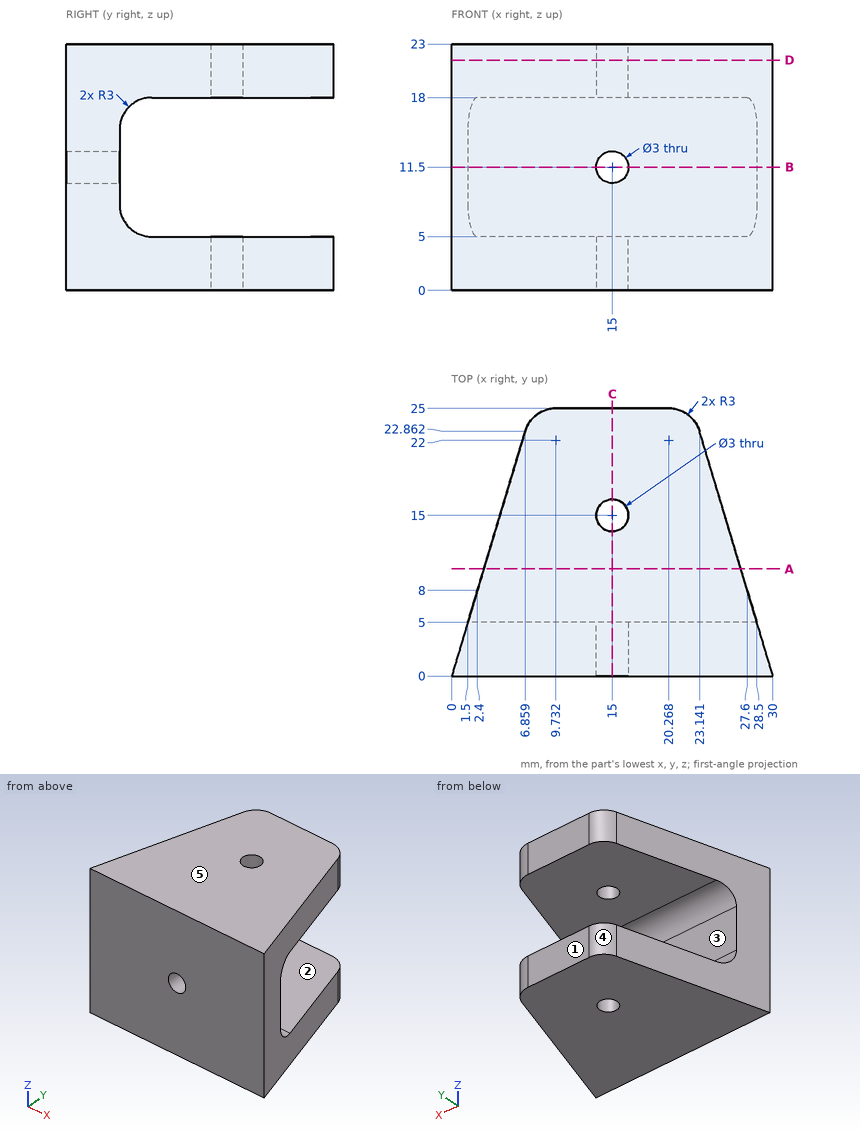
Answer from the drawing. Dimensions are ordinates in mm from the lowest x, y and z of the part. A direction names the side the tool comes from. Round coordinates to 2 decimals unless told otherwise and drop trailing zeros. Loops run counter-clockwise (first coordinate to the right, second up) from the corner with the lowest first, then second, coordinate; pieces in that order, holes last.
1) For the marked faces 1 and 2, determine the directions among +Z, -Z, +X, -X, +Y, -Y from which every point of the face is accessible in a straight line to the end or side of a thin tool.
Outcome:
face 1: +Z, -Z, +X, -X, +Y
face 2: +X, -X, +Y
2) Consider line 1 (Z direction, x = 8.5, y = 23.5); line 2 (Y direction, x = 15, z = 2.3); line 3 (Y direction, x = 14.25, z = 13). Determine where each line is inside the solid, lowest interval first.
Outcome:
line 1: z = 0 to 5, 18 to 23
line 2: y = 0 to 13.5, 16.5 to 25
line 3: y = 0 to 5
3) A cutting plane is placed at B-B on z = 11.5. Determine the outline of the cut face in (x, y).
Outcome:
outline: (0, 0) - (13.5, 0) - (13.5, 5) - (1.5, 5) - close; (16.5, 0) - (30, 0) - (28.5, 5) - (16.5, 5) - close
4) Given P1, Ø2.5, axis at x = 15, y = 15, coming from the -Z side; P2, Ø4, axis at y = 8.5, z = 18, coming from the -X side; P3, Ø1, axis at x = 11.5, z = 11.5, coming from the -Y side; P4, Ø3.5, axis at x = 12.5, z = 13, coming from the +Y side, each flat-ended and moving along its own axis, determine where each tip first touches the part or whether it passes through.
Outcome:
P1: passes through
P2: stops at x = 1.95
P3: stops at y = 0
P4: stops at y = 5
5) A cutting plane is placed at A-A on y = 10. Determine the outline of the cut face in (x, z), plus the area to 3 significant figures.
Outcome:
outline: (3, 0) - (27, 0) - (27, 5) - (3, 5) - close; (3, 18) - (27, 18) - (27, 23) - (3, 23) - close
area: 240 mm2
6) A cutting plane is placed at D-D on z = 21.5. Determine the outline of the cut face in (x, y).
Outcome:
outline: (0, 0) - (30, 0) - (23.14, 22.86) arc R3 ccw to (20.27, 25) - (9.73, 25) arc R3 ccw to (6.86, 22.86) - close; hole circle Ø3 at (15, 15)
7) For a pull along Z with two mould halves and no side action, classify the marked faces 3, 4 and 5 as released by +Z, released by -Z, zero draft, split by the parting line, or undercut.
Outcome:
face 3: undercut
face 4: zero draft
face 5: released by +Z
8) A cutting plane is placed at C-C on x = 15. Determine the outline of the cut face in (y, z).
Outcome:
outline: (0, 0) - (13.5, 0) - (13.5, 5) - (8, 5) arc R3 cw to (5, 8) - (5, 10) - (0, 10) - close; (0, 13) - (5, 13) - (5, 15) arc R3 cw to (8, 18) - (13.5, 18) - (13.5, 23) - (0, 23) - close; (16.5, 0) - (25, 0) - (25, 5) - (16.5, 5) - close; (16.5, 18) - (25, 18) - (25, 23) - (16.5, 23) - close
